Input: part model. Units: mm. Frame: model coordinates. Face numbers are marked on the shaded views. A direction names the side the tool comes from. Coordinates: 2 decimals unless noted, no trailing zeros. Write each loop counter-clockwise with the first axis right and the second up, starting at its lowest first coordinate (ties: lowest second). Pieces come first, ordered by that corner, then holes. Notation, with made-up numbers: (85, 54) -> (95, 54) arc R35 ccw to (95, 86) -> close; hole circle Ø8 at (29.5, 67). An arc over 180 degrees is marked (long way). Use one line per item in the form item = value. Start each with the question number.
(1) Cut plane C-C on y = -24.5. Return the cut outline in (x, z), plus the area to 3 significant figures.
(2) Ray query, line 1 along Y through (x, z) = (16.5, -138.5) (3 decimals); line 2 along X through (y, z) = (-13.5, -140); line 3 along Y through (x, z) = (222, -22) (3 decimals). Return the intervals inside material, ascending.
(3) Set-up query: the marked faces 1 and 2. Return all of +Z, -Z, +X, -X, +Y, -Y with unobstructed straight access to the full face (end or side cutting, diameter ignored); none if empty.
(4) Cut plane A-A on z = -137. State how many separate pieces and enclosed holes the cut face has, plus the area to 3 significant figures.
(5) Pull-direction query (X, two-part tool) for the marked faces 3, 4, 5 and 6; classes: released by +X, released by -X, zero draft, split by the parting line, or undercut.
(6) First-contact query: pin 1 (10 mm diameter, centred on x = 190, z = -59.5, fed in from +Y); pin 2 (6 mm diameter, centred on x = 132, y = -57.5, fed in from -Z); pin 3 (4.5 mm diameter, centred on y = 0, z = -154.051, fed in from +X); pin 4 (1.6 mm diameter, centred on x = 225, z = -152.5, fed in from -Y) (3 decimals). Flat tips, straight axial feed; report the tip coordinate or a pass-through.
```python
from build123d import *

# Parameters (mm, degrees)
SKETCH1_W               = 276.225
SKETCH1_H               = 152.4
BULK_EXTRUDE_DEPTH      = 136.525
SKETCH1_13_W            = 273.177
SKETCH1_13_H            = 149.352
SKETCH1_13_W_2          = 245.745
SKETCH1_13_H_2          = 1.524
INNER_SHELL_CUT_DEPTH   = 120.65
SKETCH1_14_W            = 245.745
SKETCH1_14_H            = 1.524
TOP_WALL_EXTRUDE_DEPTH  = 15.24
TOP_START               = -15.24
SKETCH1_15_W            = 273.177
SKETCH1_15_H            = 149.352
TOP_FLOOR_EXTRUDE_DEPTH = 1.524
SKETCH5_R               = 1.651
HINGE_EXTRUDE_DEPTH     = 82.55
SKETCH7_W               = 25.4635
SKETCH7_H               = 19.05
RAILS_EXTRUDE_DEPTH     = 125.476
SKETCH8_R               = 4.7625
CUT_EXTRUDE1_DEPTH      = 346.918113614
CUT_EXTRUDE1_DEPTH_BACK = 346.918113614


with BuildPart() as part:
    # Sketch1 → Bulk-Extrude (new body)
    with BuildSketch(Plane(origin=(0, 0, 0), x_dir=(1, 0, 0), z_dir=(0, 1, 0))):
        with Locations((136.5885, 74.676)):
            Rectangle(SKETCH1_W, SKETCH1_H)
    extrude(amount=-BULK_EXTRUDE_DEPTH)

    # Sketch1<13> → Inner Shell-Cut (cut)
    with BuildSketch(Plane(origin=(0, 0, 0), x_dir=(1, 0, 0), z_dir=(0, 1, 0))):
        with Locations((136.5885, 74.676)):
            Rectangle(SKETCH1_13_W, SKETCH1_13_H)
        with Locations((136.5885, -0.762)):
            Rectangle(SKETCH1_13_W_2, SKETCH1_13_H_2)
    extrude(amount=-INNER_SHELL_CUT_DEPTH, mode=Mode.SUBTRACT)

    # Sketch1<14> → Top Wall-Extrude (add)
    with BuildSketch(Plane(origin=(0, 0, 0), x_dir=(1, 0, 0), z_dir=(0, 1, 0))):
        with Locations((136.5885, -0.762)):
            Rectangle(SKETCH1_14_W, SKETCH1_14_H)
    extrude(amount=-TOP_WALL_EXTRUDE_DEPTH)

    # Sketch1<15> → Top Floor-Extrude (add)
    with BuildSketch(Plane(origin=(0, 0, 0), x_dir=(1, 0, 0), z_dir=(0, 1, 0)).offset(TOP_START)):
        with Locations((136.5885, 74.676)):
            Rectangle(SKETCH1_15_W, SKETCH1_15_H)
    extrude(amount=TOP_FLOOR_EXTRUDE_DEPTH)

    # Sketch5 → Hinge-Extrude (add)
    with BuildSketch(Plane(origin=(274.701, 0, 0), x_dir=(0, 0, -1), z_dir=(1, 0, 0))):
        with BuildLine():
            Line((150.876, 0), (150.876, -3.175))
            Line((150.876, -3.175), (154.051, -3.175))
            ThreePointArc((154.051, -3.175), (156.29606403, 2.24506403), (150.876, 0))
        make_face()
        with Locations((154.051, 0)):
            Circle(SKETCH5_R, mode=Mode.SUBTRACT)
    hinge_extrude = extrude(amount=-HINGE_EXTRUDE_DEPTH)

    # Mirror1: Hinge-Extrude across plane
    add(hinge_extrude.mirror(Plane(origin=(136.5885, 0, 0), x_dir=(0, 0, 1), z_dir=(1, 0, 0))))

    # Sketch7 → Rails-Extrude (add)
    with BuildSketch(Plane.XY.offset(-149.352)):
        with Locations((12.73175, -43.815)):
            Rectangle(SKETCH7_W, SKETCH7_H)
        with Locations((260.44525, -43.815)):
            Rectangle(SKETCH7_W, SKETCH7_H)
        with Locations((12.73175, -94.615)):
            Rectangle(SKETCH7_W, SKETCH7_H)
        with Locations((260.44525, -94.615)):
            Rectangle(SKETCH7_W, SKETCH7_H)
    extrude(amount=RAILS_EXTRUDE_DEPTH)

    # Sketch8 → Cut-Extrude1 (cut, two sides)
    with BuildSketch(Plane(origin=(274.701, 0, 0), x_dir=(0, 0, -1), z_dir=(1, 0, 0))) as cut_extrude1_sk:
        with Locations((11.176, -129.2098)):
            Circle(SKETCH8_R)
        with Locations((138.176, -129.2098)):
            Circle(SKETCH8_R)
    extrude(amount=CUT_EXTRUDE1_DEPTH, mode=Mode.SUBTRACT)
    extrude(cut_extrude1_sk.sketch, amount=-CUT_EXTRUDE1_DEPTH_BACK, mode=Mode.SUBTRACT)


solid = part.part
```
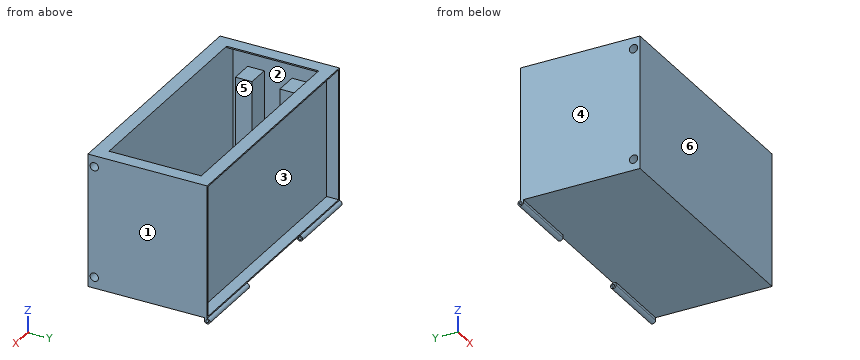
Values:
q1.outline = (-1.52, -150.88) -> (274.7, -150.88) -> (274.7, 1.52) -> (259.46, 1.52) -> (259.46, 0) -> (273.18, 0) -> (273.18, -149.35) -> (0, -149.35) -> (0, 0) -> (13.72, 0) -> (13.72, 1.52) -> (-1.52, 1.52) -> close
q1.area = 923 mm2
q2.line_1 = -136.525 to -133.961, -124.458 to -120.65, -104.14 to -85.09, -53.34 to -34.29, -15.24 to -13.716
q2.line_2 = -1.52 to 0, 273.18 to 274.7
q2.line_3 = -136.525 to -120.65, -15.24 to -13.716
q3.face_1 = +Z, -Z, +X, +Y, -Y
q3.face_2 = none
q4.separate_pieces = 2
q4.enclosed_holes = 1
q4.area = 4,560 mm2
q5.face_3 = undercut
q5.face_4 = released by -X
q5.face_5 = undercut
q5.face_6 = zero draft
q6.pin_1 = -13.72
q6.pin_2 = -150.88
q6.pin_3 = 274.7
q6.pin_4 = -3.175
